Part model, mm, in its own coordinate system. Face numbers are marked on the shaded views. A direction names the side the tool comes from. Coordinates: 2 decimals unless noted, no trailing zeros. Loops run counter-clockwise (first coordinate to the right, second up) from the corner with the lowest first, then second, coordinate; pieces in that order, holes last. Notation, with made-up numbers: (87.5, -24) - (127.5, -24) arc R22 ccw to (127.5, -16) - close; hole circle Ø9 at (50, 47.25). An arc over 180 degrees is marked (long way). Use a Markdown table: item, result. Add a question column.
1. Band-saw the part on C-C, the plane y = 23. Give the cut face in (x, z) (3 decimals), plus the area to 3 significant figures.
2. Band-saw the part on A-A, the plane z = 6.35. Count the separate pieces of the cut face and the enclosed holes in it, plus the area to 3 significant figures.
3. Wall check: probe 1 along X at (y, z) = (19, 8.25) (3 decimals); probe 2 along Y at (x, z) = (-1.3, 6.35); probe 3 along Y at (x, z) = (3, 5) (3 decimals). Give the ranges that are in metal, low to high. Write a range as [from, to].
4. Drop flat-ended pins along their axis: pin 1 (4 mm diameter, centred on x = 3, z = 5, fed in from +Y); pin 2 (1 mm diameter, centred on x = 2.5, z = 10.5, fed in from -Y) (3 decimals); pin 3 (6 mm diameter, centred on x = -0.5, z = 3.5, fed in from +Y). Give the stop position or say it passes through.
5. 3-axis set-ups, long thin cutter, end or side, ignore diameter. For the marked faces 1, 2, 3, 4 and 5: which of +Z, -Z, +X, -X, +Y, -Y reach the whole face in a straight line?
6. Band-saw the part on D-D, the plane x = 17.25. Give the cut face in (y, z) (3 decimals).
7. Pull direction X, two halves, no side cores. Call the marked faces 6, 7 and 8: pulls with the +X half, pulls with the -X half, needs draft (parallel to the pull), parting line crosses it, or undercut.
from build123d import *

# Parameters (mm, degrees)
BOSS_EXTRUDE1_DEPTH = 12.7
SKETCH2_R           = 1.5875
CUT_EXTRUDE1_DEPTH  = 76.2


with BuildPart() as part:
    # Sketch1 → Boss-Extrude1 (new body)
    with BuildSketch(Plane.XY):
        with BuildLine():
            Line((0, 0), (0, 34.925))
            Line((0, 34.925), (6.35, 34.925))
            ThreePointArc((6.35, 34.925), (9.525, 38.1), (12.7, 34.925))
            Line((12.7, 34.925), (19.05, 34.925))
            Line((19.05, 34.925), (19.05, 0))
            Line((19.05, 0), (22.225, 0))
            Line((22.225, 0), (22.225, 38.1))
            Line((22.225, 38.1), (15.024261314, 38.1))
            ThreePointArc((15.024261314, 38.1), (9.525, 41.275), (4.025738686, 38.1))
            Line((4.025738686, 38.1), (-3.175, 38.1))
            Line((-3.175, 38.1), (-3.175, 0))
            Line((-3.175, 0), (0, 0))
        make_face()
    extrude(amount=BOSS_EXTRUDE1_DEPTH)

    # Sketch2 → Cut-Extrude1 (cut)
    with BuildSketch(Plane.ZY.offset(3.175)):
        with Locations((6.35, 3.81)):
            Circle(SKETCH2_R)
    extrude(amount=-CUT_EXTRUDE1_DEPTH, mode=Mode.SUBTRACT)


solid = part.part
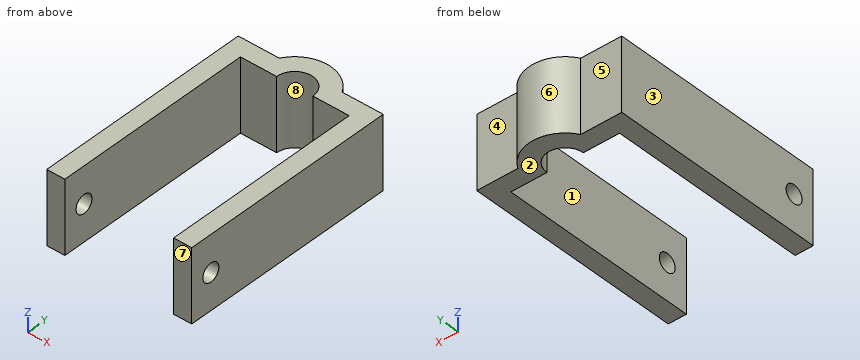
Geometry check:
| question | item | result |
|---|---|---|
| 1 | outline | (-3.175, 0) - (0, 0) - (0, 12.7) - (-3.175, 12.7) - close; (19.05, 0) - (22.225, 0) - (22.225, 12.7) - (19.05, 12.7) - close |
| 1 | area | 80.6 mm^2 |
| 2 | separate pieces | 3 |
| 2 | enclosed holes | 0 |
| 2 | area | 291 mm^2 |
| 3 | probe 1 | x = [-3.175, 0], [19.05, 22.225] |
| 3 | probe 2 | y = [0, 2.22], [5.4, 38.1] |
| 3 | probe 3 | y = [34.925, 38.1] |
| 4 | pin 1 | stops at y = 39.38 |
| 4 | pin 2 | stops at y = 34.925 |
| 4 | pin 3 | stops at y = 38.1 |
| 5 | face 1 | +Z, -Z, -Y |
| 5 | face 2 | -Z, +X, -X, +Y, -Y |
| 5 | face 3 | +Z, -Z, -X, +Y, -Y |
| 5 | face 4 | +Z, -Z, +X, +Y |
| 5 | face 5 | +Z, -Z, -X, +Y |
| 6 | outline | (34.925, 0) - (38.1, 0) - (38.1, 12.7) - (34.925, 12.7) - close |
| 7 | face 6 | parting line crosses it |
| 7 | face 7 | needs draft |
| 7 | face 8 | undercut |
